from build123d import *

# Parameters (mm, degrees)
SKETCH_1_W          = 280
SKETCH_1_H          = 280
EXTRUDE_1_DEPTH     = 150
SKETCH_2_W          = 280
SKETCH_2_H          = 272
CUT_EXTRUDE_1_DEPTH = 4
SKETCH_3_W          = 280
SKETCH_3_H          = 4
CUT_EXTRUDE_2_DEPTH = 4
SKETCH_4_W          = 270
SKETCH_4_H          = 136
CUT_EXTRUDE_3_DEPTH = 278
SKETCH_6_W          = 260
SKETCH_6_H          = 232
CUT_EXTRUDE_7_DEPTH = 247
EXTRUDE_START       = 140
SKETCH_7_W          = 1
SKETCH_7_H          = 4
EXTRUDE_2_DEPTH     = 278


with BuildPart() as part:
    # 草图1 → 凸台-拉伸1 (new body)
    with BuildSketch(Plane(origin=(0, 0, 0), x_dir=(1, 0, 0), z_dir=(0, 1, 0))):
        Rectangle(SKETCH_1_W, SKETCH_1_H)
    extrude(amount=EXTRUDE_1_DEPTH)

    # 草图2 → 切除-拉伸1 (cut)
    with BuildSketch(Plane(origin=(0, 150, 0), x_dir=(1, 0, 0), z_dir=(0, 1, 0))):
        Rectangle(SKETCH_2_W, SKETCH_2_H)
    extrude(amount=-CUT_EXTRUDE_1_DEPTH, mode=Mode.SUBTRACT)

    # 草图3 → 切除-拉伸2 (cut)
    with BuildSketch(Plane.XZ):
        with Locations((0, 138)):
            Rectangle(SKETCH_3_W, SKETCH_3_H)
        with Locations((0, -138)):
            Rectangle(SKETCH_3_W, SKETCH_3_H)
    extrude(amount=-CUT_EXTRUDE_2_DEPTH, mode=Mode.SUBTRACT)

    # 草图4 → 切除-拉伸3 (cut)
    with BuildSketch(Plane(origin=(140, 0, 0), x_dir=(0, 0, -1), z_dir=(1, 0, 0))):
        with Locations((0, 73)):
            Rectangle(SKETCH_4_W, SKETCH_4_H)
    extrude(amount=-CUT_EXTRUDE_3_DEPTH, mode=Mode.SUBTRACT)

    # 草图6 → 切除-拉伸7 (cut, through all)
    with BuildSketch(Plane(origin=(0, 146, 0), x_dir=(1, 0, 0), z_dir=(0, 1, 0))):
        with Locations((10, 0)):
            Rectangle(SKETCH_6_W, SKETCH_6_H)
    extrude(amount=-CUT_EXTRUDE_7_DEPTH, mode=Mode.SUBTRACT)

    # 草图7 → 凸台-拉伸2 (add)
    with BuildSketch(Plane(origin=(0, 0, 0), x_dir=(0, 0, -1), z_dir=(1, 0, 0)).offset(EXTRUDE_START)):
        with Locations((-134.5, 115)):
            Rectangle(SKETCH_7_W, SKETCH_7_H)
        with Locations((-134.5, 31)):
            Rectangle(SKETCH_7_W, SKETCH_7_H)
        with Locations((134.5, 31)):
            Rectangle(SKETCH_7_W, SKETCH_7_H)
        with Locations((134.5, 115)):
            Rectangle(SKETCH_7_W, SKETCH_7_H)
    extrude(amount=-EXTRUDE_2_DEPTH)


solid = part.part
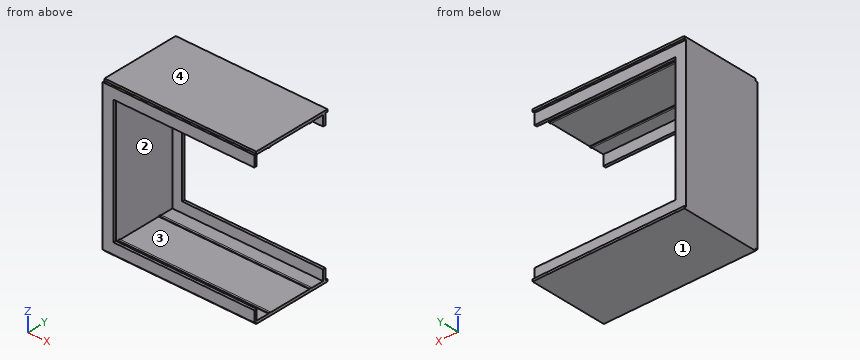
Work out the finished part from the listing and answer in its coordinate system (mm). Face numbers are marked on the shaded views. A direction names the side the tool comes from. Give positions to 0.01 mm unless a question says otherwise; leave off trailing zeros. Write each loop counter-clockwise with the first axis right and the second up, starting at its lowest first coordinate (ties: lowest second). Pieces come first, ordered by that corner, then holes. Notation, with made-up numbers: M 81,39.25 L 105,39.25 A20 cw 105,69.25 Z; hole C -32,65.25 d7. An arc over 180 degrees is marked long. Answer as CSV lines item,"result".
Q1. A tool of negligible diameter and unlimited length cuts with its end or side. For the marked faces 3 and 4, from which of +Z, -Z, +X, -X, +Y, -Y can it reach the whole face along a straight path? Write none if from no direction.
A:
face 3,"+X"
face 4,"+Z, +X, -X, +Y, -Y"
Q2. Find the intervals of material crossed by probe 1 along Z at (x, y) = (-57.5, 80); probe 2 along Y at (x, z) = (26.5, 117.5); probe 3 along X at (y, z) = (21.5, -102), in increasing order. Write a range as [from, to].
A:
probe 1,"z = [-140, -135], [135, 140]"
probe 2,"y = [0, 5], [141, 146]"
probe 3,"x = [-140, -138]"
Q3. The mould has two halves that part along Y. Classify the marked faces 1 and 2: +Y half, -Y half, draft (parallel to the pull), parting line (faces both ways), or undercut.
A:
face 1,"draft"
face 2,"undercut"
Q4. A cutting plane is placed at A-A on z = 16.5. Write down the section's boundary in (x, y).
A:
outline,"M -140,0 L -120,0 L -120,5 L -138,5 L -138,141 L -120,141 L -120,146 L -140,146 Z"
Q5. A cutting plane is placed at B-B on y = 76. Write down the section's boundary in (x, z).
A:
outline,"M -140,-140 L 140,-140 L 140,-135 L -138,-135 L -138,135 L 140,135 L 140,140 L -140,140 Z"
Q6. Given P1, Ø2, axis at y = 34.5, z = -50.5, coming from the +X side; P2, Ø1.5, axis at x = -22, y = 3.5, coming from the +Z side; P3, Ø1.1, axis at x = 39.5, z = -134.5, coming from the +Y side, each flat-ended and moving along its own axis, determine where each tip first touches the part or whether it passes through.
A:
P1,"stops at x = -138"
P2,"stops at z = 140"
P3,"stops at y = 146"
